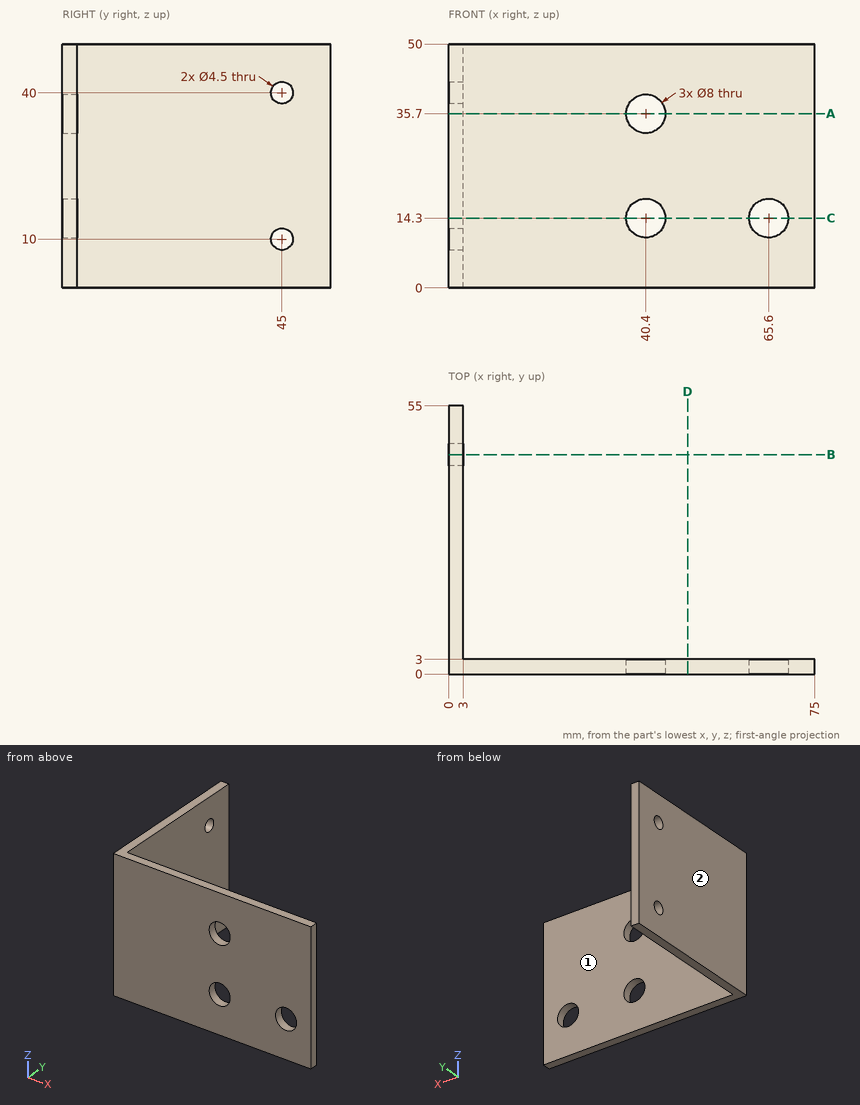
Print and shaded views of the part. All mm, measured from the part's lowest x, y and z. A direction names the side the tool comes from. Give positions to 0.01 mm unless a question says otherwise; leave off trailing zeros. Write each loop counter-clockwise with the first axis right and the second up, starting at its lowest first coordinate (ties: lowest second). Pieces come first, ordered by that corner, then holes. Notation, with made-up numbers: (-38.75, 46) - (-27.75, 46) arc R15 ccw to (-27.75, 67) - close; hole circle Ø8 at (0.25, 13). An arc over 180 degrees is marked (long way). Put each result on its own line as item: value.
(1) Tool access for the marked faces 1 and 2: list every direction of +Z, -Z, +X, -X, +Y, -Y with a clear straight run to the whole face (end or side of a thin tool).
Working result:
face 1: +Z, -Z, +X, +Y
face 2: +Z, -Z, -X, +Y, -Y
(2) Drop flat-ended pins along their axis: pin 1 Ø25 at (y, z) = (33, 27.5) entering from +X; pin 2 Ø4 at (y, z) = (45, 40) entering from -X; pin 3 Ø13 at (x, z) = (65.6, 14.3) entering from +Y. Give the stop position or say it passes through.
Working result:
pin 1: x = 3
pin 2: through
pin 3: y = 3
(3) Saw through at C-C (z = 14.3). List the corners of the cut face in (x, y).
Working result:
outline: (0, 0) - (36.4, 0) - (36.4, 3) - (3, 3) - (3, 55) - (0, 55) - close; (44.4, 0) - (61.6, 0) - (61.6, 3) - (44.4, 3) - close; (69.6, 0) - (75, 0) - (75, 3) - (69.6, 3) - close
(4) Saw through at D-D (x = 49). List the corners of the cut face in (y, z).
Working result:
outline: (0, 0) - (3, 0) - (3, 50) - (0, 50) - close
(5) Saw through at A-A (z = 35.7). List the corners of the cut face in (x, y).
Working result:
outline: (0, 0) - (36.4, 0) - (36.4, 3) - (3, 3) - (3, 55) - (0, 55) - close; (44.4, 0) - (75, 0) - (75, 3) - (44.4, 3) - close
(6) Saw through at B-B (y = 45). List the corners of the cut face in (x, z), then the cut area to 3 significant figures.
Working result:
outline: (0, 0) - (3, 0) - (3, 7.75) - (0, 7.75) - close; (0, 12.25) - (3, 12.25) - (3, 37.75) - (0, 37.75) - close; (0, 42.25) - (3, 42.25) - (3, 50) - (0, 50) - close
area: 123 mm^2
(7) Wall check: L1, parallel to X at y = 0.95, z = 14.3; L2, parallel to Z at x = 40.4, y = 1.3; L3, parallel to Y at x = 1, z = 10. Give the ranges that are in metal, low to high.
Working result:
L1: 0 to 36.4, 44.4 to 61.6, 69.6 to 75
L2: 0 to 10.3, 18.3 to 31.7, 39.7 to 50
L3: 0 to 42.75, 47.25 to 55
